Work out the finished part from the listing and answer in its coordinate system (mm). Coordinates: 2 decimals unless noted, no trailing zeros. Order: outer loops, then holes, each group sorted by start corner. A loop starts at its lowest first (then second) coordinate and runs counter-clockwise, first axis right, second up. Notation, with made-up numbers: (31, -11) - (43, -11) arc R23 ccw to (43, -2) - close; hole circle Ø3 at (36.5, -1.75). An arc over 180 degrees is marked (long way). Use CSV: the item, a comma, the result in double quotes. Start each with the question number.
from build123d import *

# Parameters (mm, degrees)
SKETCH1_W           = 10
SKETCH1_H           = 4
BOSS_EXTRUDE1_DEPTH = 16
SKETCH2_R           = 2
CUT_EXTRUDE1_DEPTH  = 5


with BuildPart() as part:
    # Sketch1 → Boss-Extrude1 (new body)
    with BuildSketch(Plane(origin=(0, 0, 0), x_dir=(1, 0, 0), z_dir=(0, 1, 0))):
        with Locations((-5, 2)):
            Rectangle(SKETCH1_W, SKETCH1_H)
    extrude(amount=BOSS_EXTRUDE1_DEPTH)

    # Sketch2 → Cut-Extrude1 (cut, through all)
    with BuildSketch(Plane.XY):
        with Locations((-5, 5)):
            Circle(SKETCH2_R)
    extrude(amount=-CUT_EXTRUDE1_DEPTH, mode=Mode.SUBTRACT)


solid = part.part
1) The part is cut by section C-C on z = -3.1. Determine the outline of the cut face in (x, y), plus the area to 3 significant figures.
2) The part is cut by section B-B on x = -5. Determine the outline of the cut face in (y, z), plus the area to 3 significant figures.
3) Straight lines are drawn through the part: line 1 (Y direction, x = -5, z = -2.55); line 2 (Y direction, x = -6.5, z = -1.9); line 3 (X direction, y = 5.75, z = -3.6). For each, find the intervals that lie inside material, in ascending order. Write a range as [from, to].
4) A flat-ended cylindrical pin translates along its axis: P1, Ø4, axis at x = -4.5, y = 9, coming from the +Z side. Find the tip coordinate at first contact, or state that the pin passes through.
5) For a pull along Y with two mould halves and no side action, classify faces 1 (the face through (-10, 8, -2)), 2 (the face through (-5, 16, -2)), 3 (the face through (-5, 0, -2)), 4 (the face through (-7, 5, -2)) as +Y half, -Y half, draft (parallel to the pull), parting line (faces both ways), or undercut.
6) The part is cut by section A-A on y = 5. Determine the outline of the cut face in (x, z).
Answer key:
1,outline,"(-10, 0) - (0, 0) - (0, 16) - (-10, 16) - close; hole circle Ø4 at (-5, 5)"
1,area,"147 mm^2"
2,outline,"(0, -4) - (3, -4) - (3, 0) - (0, 0) - close; (7, -4) - (16, -4) - (16, 0) - (7, 0) - close"
2,area,"48.0 mm^2"
3,line 1,"[0, 3], [7, 16]"
3,line 2,"[0, 3.68], [6.32, 16]"
3,line 3,"[-10, -6.85], [-3.15, 0]"
4,P1,"z = 0"
5,face 1,"draft"
5,face 2,"+Y half"
5,face 3,"-Y half"
5,face 4,"undercut"
6,outline,"(-10, -4) - (-7, -4) - (-7, 0) - (-10, 0) - close; (-3, -4) - (0, -4) - (0, 0) - (-3, 0) - close"
